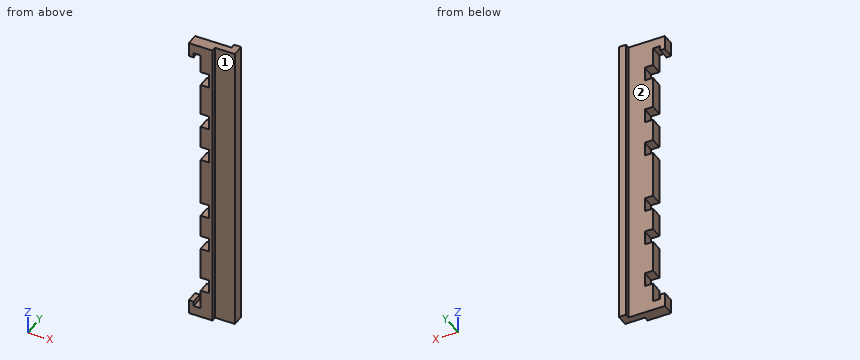
Autodesk Inventor part; units mm, degrees
ref_plane "YZ Plane" through (0, 0, 0) normal (1, 0, 0) x (0, 1, 0)
ref_plane "XZ Plane" through (0, 0, 0) normal (0, 1, 0) x (-1, 0, 0)
ref_plane "XY Plane" through (0, 0, 0) normal (0, 0, 1) x (1, 0, 0)
sketch "Sketch1" plane through (0, 0, 0) normal (1, 0, 0) x (0, 1, 0)
  line L0 (4.9903, 62.7832) -> (9.9903, 62.7832)
  line L1 (9.9903, 62.7832) -> (9.9903, -63.2168)
  line L2 (9.9903, -63.2168) -> (4.9903, -63.2168)
  line L3 (4.9903, -63.2168) -> (4.9903, 62.7832)
  point P0 (0, 0)
  dimension "d0" = 126
  dimension "d1" = 5
extrude "Extrusion1" add sketch "Sketch1" along normal blind 5
sketch "Sketch2" plane through (0, 0, 0) normal (-1, 0, 0) x (0, 0, 1)
  line L0 (-63.2168, 9.9903) -> (62.7832, 9.9903)
  line L1 (62.7832, 4.9903) -> (-63.2168, 4.9903)
  line L2 (62.7832, 9.9903) -> (58.7832, 9.9903)
  line L3 (58.7832, 9.9903) -> (58.7832, 4.9903)
  line L4 (58.7832, 4.9903) -> (62.7832, 4.9903)
  line L5 (62.7832, 4.9903) -> (62.7832, 9.9903)
  line L6 (-63.2168, 4.9903) -> (-63.2168, 9.9903)
  line L7 (-63.2168, 9.9903) -> (-59.2168, 9.9903)
  line L8 (-59.2168, 9.9903) -> (-59.2168, 4.9903)
  line L9 (-59.2168, 4.9903) -> (-63.2168, 4.9903)
  line L10 (-63.2168, 4.9903) -> (-63.2168, 9.9903)
  point P0 (0, 0)
  dimension "d4" = 4
  dimension "d5" = 4
extrude "Extrusion2" add sketch "Sketch2" along normal blind 5 contours L0 L8 L1 L6 | L0 L5 L1 L3
sketch "Sketch3" plane through (5, 9.9903, 62.7832) normal (0, 1, 0) x (1, 0, 0)
  line L0 (-10, 4) -> (-10, 0)
  line L1 (-10, 4) -> (-8, 4)
  line L2 (-8, 4) -> (-8, 6)
  line L3 (-8, 6) -> (-10, 6)
  line L4 (-10, 6) -> (-10, 4)
  line L5 (-10, 122) -> (-10, 126)
  line L6 (-10, 122) -> (-8, 122)
  line L7 (-8, 122) -> (-8, 120)
  line L8 (-8, 120) -> (-10, 120)
  line L9 (-10, 120) -> (-10, 122)
  point P0 (-5, 62.7832)
  dimension "d8" = 2
  dimension "d9" = 2
  dimension "d37" = 2
extrude "Extrusion3" add sketch "Sketch3" against normal blind 5
sketch "Sketch4" plane through (5, 4.9903, -63.2168) normal (0, 0, -1) x (-1, 0, 0)
  line L0 (10, 5) -> (0, 5)
  line L1 (0, 5) -> (-5.3853, 5)
  line L2 (-5.3853, 5) -> (-5.3853, 7)
  line L3 (-5.3853, 7) -> (-8.3853, 7)
  line L4 (-8.3853, 7) -> (-8.3853, 2)
  line L5 (-8.3853, 2) -> (0, 2)
  line L6 (0, 0) -> (0, 5)
  line L7 (0, 5) -> (0, 2)
  point P0 (5, -4.9903)
  dimension "d12" = 3
  dimension "d13" = 3
  dimension "d14" = 2
  dimension "d15" = 5
extrude "Extrusion4" add sketch "Sketch4" against normal up to surface (126 mm away)
sketch "Sketch5" plane through (0, 9.9903, 58.7832) normal (0, 1, 0) x (1, 0, 0)
  line L0 (-4.4204, 27.2832) -> (3.5, 27.2832)
  line L1 (3.5, 27.2832) -> (3.5, 33.2832)
  line L2 (3.5, 33.2832) -> (-4.4204, 33.2832)
  line L3 (-4.4204, 33.2832) -> (-4.4204, 27.2832)
  line L4 (-4.4204, 84.2832) -> (3.5, 84.2832)
  line L5 (3.5, 84.2832) -> (3.5, 90.2832)
  line L6 (3.5, 90.2832) -> (-4.4204, 90.2832)
  line L7 (-4.4204, 90.2832) -> (-4.4204, 84.2832)
  line L8 (10.3853, 122) -> (10.3853, -4)
  line L9 (-4.4204, 7.7832) -> (3.5, 7.7832)
  line L10 (3.5, 7.7832) -> (3.5, 13.7832)
  line L11 (3.5, 13.7832) -> (-4.4204, 13.7832)
  line L12 (-4.4204, 13.7832) -> (-4.4204, 7.7832)
  line L13 (-4.4204, 103.7832) -> (3.5, 103.7832)
  line L14 (3.5, 103.7832) -> (3.5, 109.7832)
  line L15 (3.5, 109.7832) -> (-4.4204, 109.7832)
  line L16 (-4.4204, 109.7832) -> (-4.4204, 103.7832)
  line L17 (0, 118) -> (0, 0)
  line L18 (-4.4204, 42.7832) -> (3.5, 42.7832)
  line L19 (3.5, 42.7832) -> (3.5, 48.7832)
  line L20 (3.5, 48.7832) -> (-4.4204, 48.7832)
  line L21 (-4.4204, 48.7832) -> (-4.4204, 42.7832)
  line L22 (-4.4204, 68.7832) -> (3.5, 68.7832)
  line L23 (3.5, 68.7832) -> (3.5, 74.7832)
  line L24 (3.5, 74.7832) -> (-4.4204, 74.7832)
  line L25 (-4.4204, 74.7832) -> (-4.4204, 68.7832)
  point P0 (0, 58.7832)
  dimension "d18" = 6
  dimension "d20" = 6
  dimension "d21" = 25.5
  dimension "d22" = 25.5
  dimension "d25" = 6
  dimension "d26" = 6
  dimension "d27" = 45
  dimension "d28" = 45
  dimension "d31" = 3.5
  dimension "d32" = 3.5
  dimension "d33" = 6
  dimension "d34" = 6
  dimension "d35" = 10
  dimension "d36" = 10
extrude "Extrusion5" cut sketch "Sketch5" against normal blind 10
properties part number "scratcher"
The listing builds one solid part. Answer for the finished solid, in the listing's coordinates (mm). Face numbers are marked on the shaded views. A direction names the side the tool comes from. Coordinates: 2 decimals unless noted, no trailing zeros. Write each loop counter-clockwise with the first axis right and the second up, starting at its lowest first coordinate (ties: lowest second). Pieces come first, ordered by that corner, then holes. Notation, with made-up numbers: (68.25, 33) - (81.25, 33) arc R17 cw to (81.25, 43) - close; hole circle Ø2 at (0, 13). An arc over 180 degrees is marked (long way). Return JSON: item names as keys, results as strings. Group by question number.
Q1. Which of the six approach directions +Z, -Z, +X, -X, +Y, -Y give full straight-line access (tool end or side, diameter ignored) to the marked faces 1 and 2?
Q2. Flat-ended cylindrical pins translate along their axes: pin 1 Ø7.5 at (x, z) = (-0.5, 25) entering from +Y; pin 2 Ø1.5 at (y, z) = (7.5, -23) entering from -X; pin 3 Ø4 at (y, z) = (6.5, 47.5) entering from -X; pin 4 Ø1.5 at (y, z) = (7, -56.5) entering from -X. Find the tip coordinate at first contact, or state that the pin passes through.
Q3. The part is cut by section A-A on z = -28. Write down the section's boundary in (x, y), and give its area (3 significant figures).
Q4. The part is cut by section B-B on x = 8.5. Write down the section's boundary in (y, z).
Q5. Find the intervals of material crossed by line 1 along X through (y, z) = (9.75, -57.5); line 2 along Y through (x, z) = (6.5, 44); line 3 along Y through (x, z) = (10.75, 34), in increasing order. Write a range as [from, to].
Q6. The part is cut by section C-C on z = 7.5. Write down the section's boundary in (x, y).
Evaluation:
{
 "1": {"face 1": "+Z, -Z, +X, -Y", "face 2": "+Z, -Z, -X, +Y"},
 "2": {"pin 1": "stops at y = 9.99", "pin 2": "stops at x = 0", "pin 3": "stops at x = 3.5", "pin 4": "stops at x = -5"},
 "3": {"outline": "(3.5, 4.99) - (5, 4.99) - (5, 6.99) - (13.39, 6.99) - (13.39, 11.99) - (10.39, 11.99) - (10.39, 9.99) - (3.5, 9.99) - close", "area": "38.7 mm2"},
 "4": {"outline": "(6.99, -63.22) - (9.99, -63.22) - (9.99, 62.78) - (6.99, 62.78) - close"},
 "5": {"line 1": "x = [-5, -3], [0, 13.39]", "line 2": "y = [6.99, 9.99]", "line 3": "y = [6.99, 11.99]"},
 "6": {"outline": "(0, 4.99) - (5, 4.99) - (5, 6.99) - (13.39, 6.99) - (13.39, 11.99) - (10.39, 11.99) - (10.39, 9.99) - (0, 9.99) - close"}
}
